Can you work these out from the drawing? Everything is in mm from the part's minimum corner. Coordinates: 2 decimals unless noted, no trailing zeros. Order: outer loops, then holes, each group sorted by start corner. A loop starts at its lowest first (then second) coordinate and runs counter-clockwise, first axis right, second up. Notation, with made-up numbers: (73, 52) -> (102, 52) arc R17 ccw to (102, 83) -> close; hole circle Ø7 at (20, 3). An arc over 180 degrees is marked (long way). Use a Markdown table: item, result. Add a question column.
1) Will these pins go through, and if not, where does the flat tip stop? pin 1 Ø1 at (x, y) = (26.5, 3.5) entering from +Z; pin 2 Ø1.5 at (x, z) = (15, 25.5) entering from +Y; pin 3 Ø2 at (x, y) = (3, 4.5) entering from -Z; pin 4 Ø7 at (x, z) = (15, 15) entering from +Y.
2) If we section it at B-B (x = 15): Write out the boundary of the cut face in (y, z).
3) If we section it at C-C (z = 26.75): Write out the boundary of the cut face in (x, y), plus the area to 3 significant figures.
4) If I drill on L1, parallel to Z at x = 15, y = 1.65; L2, parallel to X at y = 0.6, z = 11.75, over which ranges is the centre line in solid material (lowest first)? Write a range as [from, to].
5) If we section it at D-D (y = 4.8): Write out the boundary of the cut face in (x, z).
6) Thinking about a two-plate mould opening in X: for the marked faces 1, 2, 3 and 4, which applies, +X half, -X half, draft (parallel to the pull), parting line (faces both ways), or undercut?
7) If we section it at A-A (z = 15): Write out the boundary of the cut face in (x, y), plus the area to 3 significant figures.
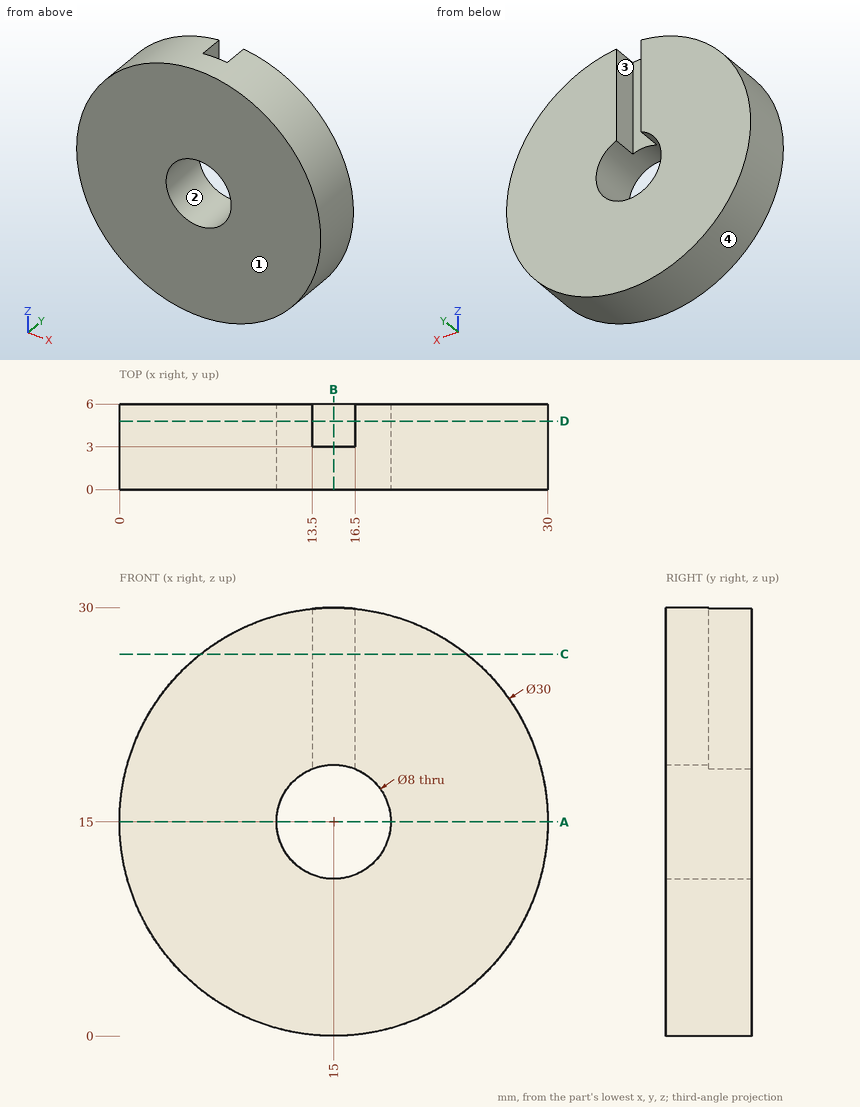
Answer sheet:
| question | item | result |
|---|---|---|
| 1 | pin 1 | z = 25.2 |
| 1 | pin 2 | y = 3 |
| 1 | pin 3 | z = 4.8 |
| 1 | pin 4 | through |
| 2 | outline | (0, 0) -> (6, 0) -> (6, 11) -> (0, 11) -> close; (0, 19) -> (3, 19) -> (3, 30) -> (0, 30) -> close |
| 3 | outline | (5.68, 0) -> (24.32, 0) -> (24.32, 6) -> (16.5, 6) -> (16.5, 3) -> (13.5, 3) -> (13.5, 6) -> (5.68, 6) -> close |
| 3 | area | 103 mm2 |
| 4 | L1 | [0, 11], [19, 30] |
| 4 | L2 | [0.36, 12.67], [17.33, 29.64] |
| 5 | outline | (13.5, 18.71) -> (13.5, 29.92) arc R15 ccw (long way) to (16.5, 29.92) -> (16.5, 18.71) arc R4 cw (long way) to start |
| 6 | face 1 | draft |
| 6 | face 2 | undercut |
| 6 | face 3 | undercut |
| 6 | face 4 | parting line |
| 7 | outline | (0, 0) -> (11, 0) -> (11, 6) -> (0, 6) -> close; (19, 0) -> (30, 0) -> (30, 6) -> (19, 6) -> close |
| 7 | area | 132 mm2 |
